Read the model definition and answer for the solid it produces. Units are mm, in the model's axes. A direction names the side the tool comes from. Coordinates: 2 decimals unless noted, no trailing zeros. Loops run counter-clockwise (first coordinate to the right, second up) from the corner with the lowest first, then second, coordinate; pieces in that order, holes last. Notation, with made-up numbers: M 65,21.5 L 99,21.5 A19 cw 99,36.5 Z; hole C 13,73 d6. An arc over 180 degrees is marked long. One line per item, written item: value. Start each with the question number.
1. The part is cut by section C-C (y = 1.25). Write down the section's boundary in (x, z), then the cut area to 3 significant figures.
2. The part is cut by section D-D (x = -30.5). Write down the section's boundary in (y, z).
3. The part is cut by section A-A (y = 11.25). Write down the section's boundary in (x, z), then the cut area to 3 significant figures.
4. The part is cut by section B-B (z = 20). Write down the section's boundary in (x, y).
5. For faces 5 (the face through (47, 17, 27)), 6 (the face through (44.25, 17, 0)), 7 (the face through (-51, 5, -26)), determine the directions among +Z, -Z, +X, -X, +Y, -Y from which every point of the face is accessible in a straight line to the end or side of a thin tool.
6. Flat-ended cylindrical pins translate along their axes: pin 1 (5 mm diameter, centred on x = 41, z = 20.5, fed in from -Y); pin 2 (3 mm diameter, centred on y = -2.5, z = -7.5, fed in from +X); pin 3 (1 mm diameter, centred on y = -7, z = -18.5, fed in from -X). Find the tip coordinate at first contact, or state that the pin passes through.
7. Consider probe 1 along X at (y, z) = (11, 20); probe 2 along X at (y, z) = (11.5, -21); probe 3 along X at (y, z) = (2.4, -7.5). Determine where each line is inside the solid, lowest interval first.
8. Determine the mould class of faces 1 (the face through (-49.75, 17, 0)), 2 (the face through (-47, 17, -27)), 3 (the face through (-1, 0, 12)), 4 (the face through (-47, 17, 27)) for opening direction X: +X half, -X half, draft (parallel to the pull), parting line (faces both ways), or undercut.
```python
from build123d import *

# Parameters (mm, degrees)
SKETCH1_W           = 104
SKETCH1_H           = 55
BOSS_EXTRUDE1_DEPTH = 5
BOSS_EXTRUDE2_DEPTH = 11
BOSS_EXTRUDE3_DEPTH = 2
SKETCH4_R           = 1.9
CUT_EXTRUDE1_DEPTH  = 23
SKETCH5_R           = 17.25
SKETCH5_R_2         = 12.75
BOSS_EXTRUDE4_DEPTH = 10
SKETCH7_R           = 7.5
CUT_EXTRUDE2_DEPTH  = 35


with BuildPart() as part:
    # Sketch1 → Boss-Extrude1 (new body)
    with BuildSketch(Plane(origin=(0, 0, 0), x_dir=(1, 0, 0), z_dir=(0, 1, 0))):
        Rectangle(SKETCH1_W, SKETCH1_H)
    extrude(amount=BOSS_EXTRUDE1_DEPTH)

    # Sketch2 → Boss-Extrude2 (add)
    with BuildSketch(Plane(origin=(0, 5, 0), x_dir=(1, 0, 0), z_dir=(0, 1, 0))):
        with BuildLine():
            Line((-52, -22.5), (-52, 22.5))
            ThreePointArc((-52, 22.5), (-47, 27.5), (-42, 22.5))
            Line((-42, 22.5), (-42, -22.5))
            ThreePointArc((-42, -22.5), (-47, -27.5), (-52, -22.5))
        make_face()
        with BuildLine():
            Line((42, -22.5), (42, 22.5))
            ThreePointArc((42, 22.5), (47, 27.5), (52, 22.5))
            Line((52, 22.5), (52, -22.5))
            ThreePointArc((52, -22.5), (47, -27.5), (42, -22.5))
        make_face()
    extrude(amount=BOSS_EXTRUDE2_DEPTH)

    # Sketch3 → Boss-Extrude3 (add)
    with BuildSketch(Plane(origin=(0, 16, 0), x_dir=(1, 0, 0), z_dir=(0, 1, 0))):
        with BuildLine():
            Line((-49.75, -24.25), (-49.75, 24.25))
            ThreePointArc((-49.75, 24.25), (-47, 27), (-44.25, 24.25))
            Line((-44.25, 24.25), (-44.25, -24.25))
            ThreePointArc((-44.25, -24.25), (-47, -27), (-49.75, -24.25))
        make_face()
        with BuildLine():
            Line((44.25, -24.25), (44.25, 24.25))
            ThreePointArc((44.25, 24.25), (47, 27), (49.75, 24.25))
            Line((49.75, 24.25), (49.75, -24.25))
            ThreePointArc((49.75, -24.25), (47, -27), (44.25, -24.25))
        make_face()
    extrude(amount=BOSS_EXTRUDE3_DEPTH)

    # Sketch4 → Cut-Extrude1 (cut)
    with BuildSketch(Plane(origin=(0, 18, 0), x_dir=(1, 0, 0), z_dir=(0, 1, 0))):
        with Locations(Location((-47, 0, 0), (0, 0, 270))):
            Circle(SKETCH4_R)
        with Locations(Location((-47, 20, 0), (0, 0, 270))):
            Circle(SKETCH4_R)
        with Locations(Location((-47, -20, 0), (0, 0, 270))):
            Circle(SKETCH4_R)
        with Locations(Location((47, 0, 0), (0, 0, 270))):
            Circle(SKETCH4_R)
        with Locations(Location((47, 20, 0), (0, 0, 270))):
            Circle(SKETCH4_R)
        with Locations(Location((47, -20, 0), (0, 0, 270))):
            Circle(SKETCH4_R)
    extrude(amount=-CUT_EXTRUDE1_DEPTH, mode=Mode.SUBTRACT)

    # Sketch5 → Boss-Extrude4 (add)
    with BuildSketch(Plane.XZ):
        with Locations(Location((0, -7.5, 0), (0, 0, 270))):
            Circle(SKETCH5_R)
        with Locations(Location((0, -7.5, 0), (0, 0, 270))):
            Circle(SKETCH5_R_2, mode=Mode.SUBTRACT)
    extrude(amount=BOSS_EXTRUDE4_DEPTH)

    # Sketch7 → Cut-Extrude2 (cut)
    with BuildSketch(Plane.XZ.offset(10)):
        with Locations(Location((0, -7.5, 0), (0, 0, 270))):
            Circle(SKETCH7_R)
    extrude(amount=-CUT_EXTRUDE2_DEPTH, mode=Mode.SUBTRACT)


solid = part.part
```
Answer block:
1. outline: M -52,-27.5 L 52,-27.5 L 52,27.5 L -52,27.5 Z; hole C -47,-20 d3.8; hole C -47,0 d3.8; hole C -47,20 d3.8; hole C 0,-7.5 d15; hole C 47,-20 d3.8; hole C 47,0 d3.8; hole C 47,20 d3.8
1. area: 5,480 mm2
2. outline: M 0,-27.5 L 5,-27.5 L 5,27.5 L 0,27.5 Z
3. outline: M -52,-22.5 A5 ccw -42,-22.5 L -42,22.5 A5 ccw -52,22.5 Z; M 42,-22.5 A5 ccw 52,-22.5 L 52,22.5 A5 ccw 42,22.5 Z; hole C -47,-20 d3.8; hole C -47,0 d3.8; hole C -47,20 d3.8; hole C 47,-20 d3.8; hole C 47,0 d3.8; hole C 47,20 d3.8
3. area: 989 mm2
4. outline: M -52,0 L -48.9,0 L -48.9,18 L -49.75,18 L -49.75,16 L -52,16 Z; M -45.1,0 L 45.1,0 L 45.1,18 L 44.25,18 L 44.25,16 L 42,16 L 42,5 L -42,5 L -42,16 L -44.25,16 L -44.25,18 L -45.1,18 Z; M 48.9,0 L 52,0 L 52,16 L 49.75,16 L 49.75,18 L 48.9,18 Z
5. face 5: +Z, +Y
5. face 6: +Z, -Z, +Y
5. face 7: -Z, -X, +Y
6. pin 1: stops at y = 0
6. pin 2: stops at x = 17.25
6. pin 3: stops at x = -13.69
7. probe 1: x = -52 to -48.9, -45.1 to -42, 42 to 45.1, 48.9 to 52
7. probe 2: x = -52 to -48.62, -45.38 to -42, 42 to 45.38, 48.62 to 52
7. probe 3: x = -52 to -7.5, 7.5 to 52
8. face 1: -X half
8. face 2: undercut
8. face 3: draft
8. face 4: undercut
